```python
from build123d import *

# Parameters (mm, degrees)
BOSS_EXTRUDE1_DEPTH             = 30.48
BOSS_EXTRUDE1_DEPTH_BACK        = 30.48
SKETCH1_R                       = 22.225
SKETCH1_R_2                     = 7.62
CUT_EXTRUDE2_DEPTH              = 76.2
BOSS_EXTRUDE3_REACH             = 447.466
SKETCH5_R                       = 7.62
BOSS_EXTRUDE3_DIRECTION_2_REACH = 447.466


with BuildPart() as part:
    # Sketch1 → Boss-Extrude1 (new, two sides: drawn at the far end of the back side and taken through both)
    with BuildSketch(Plane(origin=(0, 0, 0), x_dir=(1, 0, 0), z_dir=(0, 1, 0)).offset(-BOSS_EXTRUDE1_DEPTH_BACK)):
        with BuildLine():
            Line((359.662846674, 198.232216379), (28.235630228, 198.232216379))
            ThreePointArc((28.235630228, 198.232216379), (4.898580527, 190.2485261), (-8.658113435, 169.643350826))
            Line((-8.658113435, 169.643350826), (-37.51656391, 6.642095481))
            ThreePointArc((-37.51656391, 6.642095481), (-6.629045926, -37.518871919), (37.52117539, -6.615995569))
            Line((37.52117539, -6.615995569), (54.653846734, 90.548211948))
            ThreePointArc((54.653846734, 90.548211948), (67.684814195, 113.118509662), (92.175022124, 122.032216379))
            Line((92.175022124, 122.032216379), (359.662846674, 122.032216379))
            ThreePointArc((359.662846674, 122.032216379), (397.762846674, 160.132216379), (359.662846674, 198.232216379))
        make_face()
        with Locations(Location((0, 0, 0), (0, 0, 270))):
            Circle(SKETCH1_R, mode=Mode.SUBTRACT)
        with Locations(Location((359.662846674, 160.132216379, 0), (0, 0, 270))):
            Circle(SKETCH1_R_2, mode=Mode.SUBTRACT)
    extrude(amount=BOSS_EXTRUDE1_DEPTH + BOSS_EXTRUDE1_DEPTH_BACK)

    # Sketch4 → Cut-Extrude2 (cut)
    with BuildSketch(Plane(origin=(0, 0, -198.232216379), x_dir=(-1, 0, 0), z_dir=(0, 0, -1))):
        Polygon((-397.762846674, 0), (-397.762846674, 27.94), (-321.562846674, 27.94), (-321.562846674, -27.94), (-397.762846674, -27.94), align=None)
    extrude(amount=-CUT_EXTRUDE2_DEPTH, mode=Mode.SUBTRACT)

    # Boss-Extrude3: up to this face of the body (flat: up to its plane)
    boss_extrude3_end = Plane(part.part.faces().sort_by_distance((144.088603617, 30.48, -132.672626022))[0])
    # Sketch5 → Boss-Extrude3 (add, up to the picked face)
    with BuildSketch(Plane(origin=(0, 0, 0), x_dir=(1, 0, 0), z_dir=(0, 1, 0)), mode=Mode.PRIVATE) as boss_extrude3_sk1:
        with Locations((359.662846674, 160.132216379)):
            Circle(SKETCH5_R)
    boss_extrude3_tool1 = split(extrude(boss_extrude3_sk1.sketch, amount=BOSS_EXTRUDE3_REACH, mode=Mode.PRIVATE), bisect_by=boss_extrude3_end, keep=Keep.BOTH, mode=Mode.PRIVATE)
    add(boss_extrude3_tool1.solids().sort_by(Axis((359.662847, 0, -160.132216), (0, 1, 0)))[0])

    # Boss-Extrude3 direction 2: up to this face of the body (flat: up to its plane)
    boss_extrude3_direction_2_end = Plane(part.part.faces().sort_by_distance((144.088603617, -30.48, -132.672626022))[0])
    # Sketch5 → Boss-Extrude3 direction 2 (add, up to the picked face)
    with BuildSketch(Plane(origin=(0, 0, 0), x_dir=(1, 0, 0), z_dir=(0, 1, 0)), mode=Mode.PRIVATE) as boss_extrude3_direction_2_sk1:
        with Locations((359.662846674, 160.132216379)):
            Circle(SKETCH5_R)
    boss_extrude3_direction_2_tool1 = split(extrude(boss_extrude3_direction_2_sk1.sketch, amount=-BOSS_EXTRUDE3_DIRECTION_2_REACH, mode=Mode.PRIVATE), bisect_by=boss_extrude3_direction_2_end, keep=Keep.BOTH, mode=Mode.PRIVATE)
    add(boss_extrude3_direction_2_tool1.solids().sort_by(Axis((359.662847, 0, -160.132216), (0, -1, 0)))[0])


solid = part.part
```
The model under review builds one solid part; all positions refer to its coordinate system, in mm. A direction names the side the tool comes from. Coordinates: 2 decimals unless noted, no trailing zeros. Order: outer loops, then holes, each group sorted by start corner. A loop starts at its lowest first (then second) coordinate and runs counter-clockwise, first axis right, second up. Notation, with made-up numbers: (-24.75, 81.5) -> (13.25, 81.5) arc R24 ccw to (13.25, 91.5) -> close; hole circle Ø5 at (52.5, 75.25). An arc over 180 degrees is marked (long way). Answer in a Markdown table with one row per item. Add a question column.
Item 1: We need section B-B on y = -21.5. Write out the cut boundary in (x, z) (3 decimals).
Item 2: Clearance check with flat-ended pins moving along their axes: pin 1 (8 mm diameter, centred on y = 20.5, z = -1, fed in from +X); pin 2 (12 mm diameter, centred on y = 14.5, z = 6.5, fed in from +X); pin 3 (10 mm diameter, centred on y = 10, z = -131, fed in from -X). State where each tip first meets the part, or that it passes through.
Item 3: Mouldability with a two-part tool opening along X and no side actions: class faces 1 (the cylindrical face through (18.74, -0.43, 11.95)), 2 (the flat face through (128, 30.48, -134)), 3 (the cylindrical face through (5.178, -0.427, -190.463)), 4 (the cylindrical face through (397.754, -29.228, -159.294)) as +X half, -X half, draft (parallel to the pull), parting line (faces both ways), or undercut.
Item 4: We need section D-D on x = 306. Write out the cut boundary in (y, z), plus the area to 3 significant figures.
Item 5: To check wall thickness, follow probe 1 along Y at (x, z) = (370, -131.5); probe 2 along Z at (x, y) = (183, -3); probe 3 along X at (y, z) = (0.5, 0) (3 decimals). State the ranges of each line that lie inside material, in increasing order.
Item 6: We need section A-A on z = 0. Write out the cut boundary in (x, y) (3 decimals).
Item 7: We need section C-C on x = 0. Write out the cut boundary in (y, z) (3 decimals), plus the area to 3 significant figures.
Item 8: Machinability: for faces 5 (the flat face through (196, 0, -198.232)), 6 (the flat face through (194, 0, -122.032)), which of the approach directions +Z, -Z, +X, -X, +Y, -Y give a long, thin tool a straight path to every point of the face, cutting with its end or side? Answer none if there is none.
Final values:
| question | item | result |
|---|---|---|
| 1 | outline | (-37.517, -6.642) -> (-8.658, -169.643) arc R38.1 ccw to (28.236, -198.232) -> (321.563, -198.232) -> (321.563, -122.032) -> (92.175, -122.032) arc R38.1 cw to (54.654, -90.548) -> (37.521, 6.616) arc R38.1 ccw to start; circle Ø15.24 at (359.663, -160.132); hole circle Ø44.45 at (0, 0) |
| 2 | pin 1 | stops at x = 39.57 |
| 2 | pin 2 | stops at x = 38.6 |
| 2 | pin 3 | stops at x = -16.38 |
| 3 | face 1 | undercut |
| 3 | face 2 | draft |
| 3 | face 3 | -X half |
| 3 | face 4 | +X half |
| 4 | outline | (-30.48, -198.23) -> (30.48, -198.23) -> (30.48, -122.03) -> (-30.48, -122.03) -> close |
| 4 | area | 4,650 mm2 |
| 5 | probe 1 | y = -30.48 to -27.94, 27.94 to 30.48 |
| 5 | probe 2 | z = -198.23 to -122.03 |
| 5 | probe 3 | x = -38.1 to -22.225, 22.225 to 38.688 |
| 6 | outline | (-38.1, -30.48) -> (-22.225, -30.48) -> (-22.225, 30.48) -> (-38.1, 30.48) -> close; (22.225, -30.48) -> (38.688, -30.48) -> (38.688, 30.48) -> (22.225, 30.48) -> close |
| 7 | outline | (-30.48, -185.713) -> (30.48, -185.713) -> (30.48, -22.225) -> (-30.48, -22.225) -> close; (-30.48, 22.225) -> (30.48, 22.225) -> (30.48, 38.1) -> (-30.48, 38.1) -> close |
| 7 | area | 10,900 mm2 |
| 8 | face 5 | -Z, +X, -X, +Y, -Y |
| 8 | face 6 | +Z, +X, +Y, -Y |
